```python
from build123d import *

# Parameters (mm, degrees)
F1_DEPTH = 63.5
F2_DEPTH = 25.4
F3_DEPTH = 7.9375
F4_R     = 5.08


with BuildPart() as f1:
    # F0 (on Front) → F1 (new body, symmetric)
    with BuildSketch(Plane.XZ):
        Polygon((28.575, 9.525), (-47.625, 9.525), (-47.625, -9.525), (47.625, -9.525), (47.625, 9.525), align=None)
    extrude(amount=F1_DEPTH, both=True)

    # F0 (on Front) → F2 (join, symmetric)
    with BuildSketch(Plane.XZ):
        with BuildLine():
            Line((28.575, 34.925), (28.575, 9.525))
            Line((28.575, 9.525), (47.625, 9.525))
            Line((47.625, 9.525), (47.625, 34.925))
            ThreePointArc((47.625, 34.925), (52.27468, 46.15032), (63.5, 50.8))
            Line((63.5, 50.8), (88.9, 50.8))
            Line((88.9, 50.8), (88.9, 69.85))
            Line((88.9, 69.85), (63.5, 69.85))
            add(Edge.make_bspline(
                [(60.686772, 69.736512), (61.617392, 69.776715), (62.555116, 69.814521), (63.5, 69.85)],
                knots=[124.561672, 124.561672, 124.561672, 124.561672, 126.443154, 126.443154, 126.443154, 126.443154], degree=3))
            ThreePointArc((60.686772, 69.736512), (37.828931, 58.605199), (28.575, 34.925))
        make_face()
    extrude(amount=F2_DEPTH, both=True)

    # F0 (on Front) → F3 (join, symmetric)
    with BuildSketch(Plane.XZ):
        with BuildLine():
            add(Edge.make_bspline(
                [(-47.625, 9.525), (-31.403715, 53.903915), (-0.924034, 67.074893), (60.686772, 69.736512)],
                knots=[0, 0, 0, 0, 124.561672, 124.561672, 124.561672, 124.561672], degree=3))
            Line((-47.625, 9.525), (28.575, 9.525))
            Line((28.575, 9.525), (28.575, 34.925))
            ThreePointArc((28.575, 34.925), (37.828931, 58.605199), (60.686772, 69.736512))
        make_face()
    extrude(amount=F3_DEPTH, both=True)

    # F4
    f4_edges = [f1.edges().sort_by_distance(p)[0] for p in [
        (-47.625, -63.5, 0),
        (47.625, -63.5, 0),
        (-47.625, 63.5, 0),
        (47.625, 63.5, 0),
    ]]
    fillet(f4_edges, radius=F4_R)


solid = f1.part
```
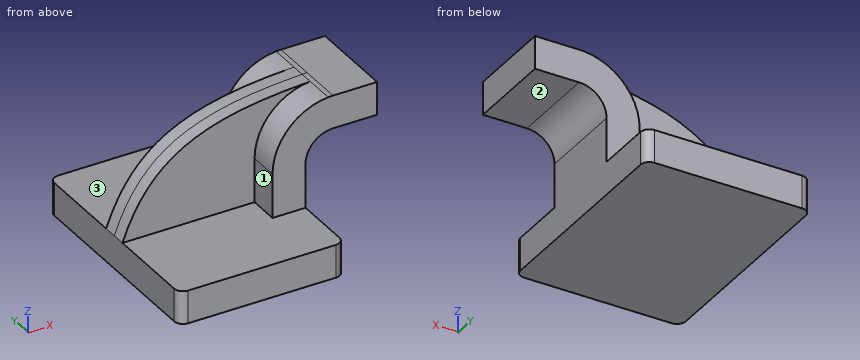
Can you work these out from the model? Positions are in its coordinate system, mm. Face numbers are marked on the shaded views. A direction names the side the tool comes from. Give positions to 0.01 mm unless a question says otherwise; leave off trailing zeros. Loops run counter-clockwise (first coordinate to the right, second up) from the corner with the lowest first, then second, coordinate; pieces in that order, holes last. Notation, with made-up numbers: M 41,42.25 L 47,42.25 A22 ccw 47,55.25 Z; hole C 55.25,-30 d5. An arc over 180 degrees is marked long. One line per question, with ' | ' between items. Start each with the question number.
Q1. If we section it at B-B (y = 54): Please give me the cut outline in (x, z) (3 decimals), plus the area to 3 significant figures.
Q2. For the marked faces 1, 2 and 3, which set-ups out of +Z, -Z, +X, -X, +Y, -Y let a thin tool reach every point of the face, with its end or its side?
Q3. If I drill on line 1 (Z direction, x = -29, y = 42) (3 decimals); line 2 (X direction, y = -44, z = 1.5) (3 decimals); line 3 (Y direction, x = 34, z = 42), over which ranges is the centre line in solid material (lowest first)? Write a range as from..to.
Q4. If we section it at A-A (z = -2.5): Please give me the cut outline in (x, y) (3 decimals).
Q5. For pin 1 Ø19 at (y, z) = (18, 28) entering from -X (3 decimals); pin 2 Ø18 at (x, z) = (44, 47) entering from +Y; pin 3 Ø2 at (x, z) = (5, 37) entering from -Y, each with a flat end and sliding along its axis, tell me the tip position at first contact or that it passes through.
Computed:
1) outline: M -47.625,-9.525 L 47.625,-9.525 L 47.625,9.525 L -47.625,9.525 Z | area: 1,810 mm²
2) face 1: +Z, -X, -Y | face 2: -Z, +X, +Y, -Y | face 3: +Z, -X, +Y
3) line 1: z = -9.525..9.525 | line 2: x = -47.625..47.625 | line 3: y = -25.4..25.4
4) outline: M -47.625,-58.42 A5.08 ccw -42.545,-63.5 L 42.545,-63.5 A5.08 ccw 47.625,-58.42 L 47.625,58.42 A5.08 ccw 42.545,63.5 L -42.545,63.5 A5.08 ccw -47.625,58.42 Z
5) pin 1: stops at x = 28.575 | pin 2: stops at y = 25.4 | pin 3: stops at y = -7.94
